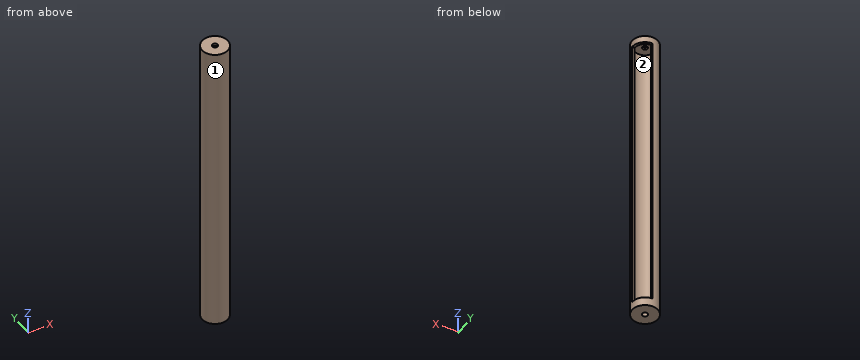
```python
from build123d import *

# Parameters (mm, degrees)
CYLINDER_R        = 7.5
CYLINDER_DEPTH    = 175
BOX_W             = 10
BOX_H             = 10
BOX_DEPTH         = 166
CYLINDER001_R     = 6
CYLINDER001_DEPTH = 171
CYLINDER002_R     = 1.55
CYLINDER002_DEPTH = 175


with BuildPart() as part:
    # Cylinder → Cylinder (join)
    with BuildSketch(Plane.XY):
        Circle(CYLINDER_R)
    extrude(amount=CYLINDER_DEPTH)

    # Box → Box (cut)
    with BuildSketch(Plane.XY.offset(5)):
        with Locations((5, 5)):
            Rectangle(BOX_W, BOX_H)
    extrude(amount=BOX_DEPTH, mode=Mode.SUBTRACT)

    # Cylinder001 → Cylinder001 (cut)
    with BuildSketch(Plane.XY.offset(2.5)):
        Circle(CYLINDER001_R)
    extrude(amount=CYLINDER001_DEPTH, mode=Mode.SUBTRACT)

    # Cylinder002 → Cylinder002 (cut)
    with BuildSketch(Plane.XY):
        Circle(CYLINDER002_R)
    extrude(amount=CYLINDER002_DEPTH, mode=Mode.SUBTRACT)


solid = part.part
```
Read the model definition and answer for the solid it produces. Units are mm, in the model's axes. Face numbers are marked on the shaded views. A direction names the side the tool comes from. Give positions to 0.01 mm unless a question says otherwise; leave off trailing zeros. Order: outer loops, then holes, each group sorted by start corner. A loop starts at its lowest first (then second) coordinate and runs counter-clockwise, first axis right, second up. Notation, with made-up numbers: (70, 10.5) -> (107, 10.5) arc R26 cw to (107, 35.5) -> close; hole circle Ø11 at (-22, 80). An arc over 180 degrees is marked (long way). One line per item, written item: value. Start each with the question number.
(1) The part is cut by section C-C (x = -3.5). Determine the outline of the cut face in (y, z), and give its area (3 significant figures).
(2) The part is cut by section D-D (z = 111). Determine the outline of the cut face in (x, y), and give its area (3 significant figures).
(3) Flat-ended cylindrical pins translate along their axes: P1, Ø1, axis at x = -1.5, z = 84.5, coming from the +Y side; P2, Ø3, axis at y = 2.5, z = 70.5, coming from the +X side; P3, Ø2.5, axis at x = 0, y = 0, coming from the +Z side; P4, Ø4, axis at x = 5.5, z = 121.5, coming from the +Y side. Find the tip coordinate at first contact, or state that the pin passes through.
(4) The part is cut by section B-B (x = 4). Determine the outline of the cut face in (y, z).
(5) A tool of negligible diameter and unlimited length cuts with its end or side. For the marked faces 1 and 2, from which of +Z, -Z, +X, -X, +Y, -Y can it reach the whole face along a straight path? Write none if from no direction.
(6) Straight lines are drawn through the part: L1, parallel to Y at x = 0, z = 0.9; L2, parallel to Z at x = 5.25, y = -2.25; L3, parallel to Y at x = -2.5, z = 52. For each, find the intervals that lie inside material, in ascending order.
(7) The part is cut by section A-A (y = -4.25). Determine the outline of the cut face in (x, z), and give its area (3 significant figures).
Taken from the geometry:
1. outline: (-6.63, 0) -> (6.63, 0) -> (6.63, 175) -> (-6.63, 175) -> close; hole (-4.87, 2.5) -> (4.87, 2.5) -> (4.87, 173.5) -> (-4.87, 173.5) -> close
1. area: 655 mm^2
2. outline: (0, 6) -> (0, 7.5) arc R7.5 ccw (long way) to (7.5, 0) -> (6, 0) arc R6 cw (long way) to start
2. area: 47.7 mm^2
3. P1: y = 7.43
3. P2: x = -4.47
3. P3: through
3. P4: y = 0
4. outline: (-6.34, 0) -> (6.34, 0) -> (6.34, 5) -> (4.47, 5) -> (4.47, 2.5) -> (-4.47, 2.5) -> (-4.47, 173.5) -> (4.47, 173.5) -> (4.47, 171) -> (6.34, 171) -> (6.34, 175) -> (-6.34, 175) -> close
5. face 1: +Z, -Z
5. face 2: none
6. L1: -7.5 to -1.55, 1.55 to 7.5
6. L2: 0 to 2.5, 173.5 to 175
6. L3: -7.07 to -5.45, 5.45 to 7.07
7. outline: (-6.18, 0) -> (6.18, 0) -> (6.18, 175) -> (-6.18, 175) -> close; hole (-4.24, 2.5) -> (4.24, 2.5) -> (4.24, 173.5) -> (-4.24, 173.5) -> close
7. area: 714 mm^2
